from build123d import *

# Parameters (mm, degrees)
SKETCH013_R     = 13
SKETCH013_R_2   = 8.5
PAD008_DEPTH    = 5
SKETCH014_R     = 12
SKETCH014_R_2   = 9.5
POCKET006_DEPTH = 0.5
SKETCH015_R     = 12
SKETCH015_R_2   = 9.5
POCKET007_DEPTH = 0.5


with BuildPart() as part:
    # Sketch013 → Pad008 (new body)
    with BuildSketch(Plane.XY):
        Circle(SKETCH013_R)
        Circle(SKETCH013_R_2, mode=Mode.SUBTRACT)
    extrude(amount=PAD008_DEPTH)

    # Sketch014 → Pocket006 (cut)
    with BuildSketch(Plane.XY.offset(5)):
        Circle(SKETCH014_R)
        Circle(SKETCH014_R_2, mode=Mode.SUBTRACT)
    extrude(amount=-POCKET006_DEPTH, mode=Mode.SUBTRACT)

    # Sketch015 → Pocket007 (cut)
    with BuildSketch(Plane.XY):
        Circle(SKETCH015_R)
        Circle(SKETCH015_R_2, mode=Mode.SUBTRACT)
    extrude(amount=POCKET007_DEPTH, mode=Mode.SUBTRACT)


solid = part.part
Geometry check sheet. Reference: the model listing, model coordinates, mm. A direction names the side the tool comes from. Give positions to 0.01 mm unless a question says otherwise; leave off trailing zeros. Order: outer loops, then holes, each group sorted by start corner. A loop starts at its lowest first (then second) coordinate and runs counter-clockwise, first axis right, second up.
1) Cross-section at C-C (z = 2.65). Record the boundary of the cut face in (x, y).
Results are:
outline: circle Ø26 at (0, 0); hole circle Ø17 at (0, 0)
2) Tool access check on faces 1 (the flat face through (9, 4, 0.5)), 2 (the flat face through (9, 4, 4.5)), 3 (the cylindrical face through (4.57, 7.167, 2.465)). Record the directions out of +Z, -Z, +X, -X, +Y, -Y that give a thin tool (end or side, any length) a straight path to the whole face; none if there is none.
Results are:
face 1: -Z
face 2: +Z
face 3: +Z, -Z
3) Cross-section at A-A (y = 0). Record the boundary of the cut face in (x, z).
Results are:
outline: (-13, 0) - (-12, 0) - (-12, 0.5) - (-9.5, 0.5) - (-9.5, 0) - (-8.5, 0) - (-8.5, 5) - (-9.5, 5) - (-9.5, 4.5) - (-12, 4.5) - (-12, 5) - (-13, 5) - close; (8.5, 0) - (9.5, 0) - (9.5, 0.5) - (12, 0.5) - (12, 0) - (13, 0) - (13, 5) - (12, 5) - (12, 4.5) - (9.5, 4.5) - (9.5, 5) - (8.5, 5) - close
4) Material ranges on probe 1 along Y at (x, z) = (0, 0.35); probe 2 along Y at (x, z) = (0, 2.85); probe 3 along X at (y, z) = (-6, 0.4), recorded low to high.
Results are:
probe 1: y = -13 to -12, -9.5 to -8.5, 8.5 to 9.5, 12 to 13
probe 2: y = -13 to -8.5, 8.5 to 13
probe 3: x = -11.53 to -10.39, -7.37 to -6.02, 6.02 to 7.37, 10.39 to 11.53
5) Gauge pin test, flat ends, axial feed: pin 1 (5 mm diameter, centred on x = -3, y = 7, fed in from +Z); pin 2 (12 mm diameter, centred on x = 1.5, y = 0, fed in from -Z); pin 3 (1 mm diameter, centred on x = -9, z = 2.5, fed in from -Y). Record the tip position at first contact, or that the pin passes through.
Results are:
pin 1: stops at z = 5
pin 2: passes through
pin 3: stops at y = -9.84
6) Cross-section at D-D (x = 11.25). Record the boundary of the cut face in (y, z).
Results are:
outline: (-6.51, 0) - (-4.18, 0) - (-4.18, 0.5) - (4.18, 0.5) - (4.18, 0) - (6.51, 0) - (6.51, 5) - (4.18, 5) - (4.18, 4.5) - (-4.18, 4.5) - (-4.18, 5) - (-6.51, 5) - close
7) Draft check along Y on faces 4 (the flat face through (9, -9, 0)), 5 (the cylindrical face through (4.38, -8.43, 0.25)), 6 (the cylindrical face through (-10.316, -7.91, 2.465)). Enter one of: released by +Y, released by -Y, zero draft, split by the parting line, or undercut.
Results are:
face 4: zero draft
face 5: undercut
face 6: split by the parting line
8) Cross-section at B-B (x = 8). Record the boundary of the cut face in (y, z), then the cut area to 3 significant figures.
Results are:
outline: (-10.25, 0) - (-8.94, 0) - (-8.94, 0.5) - (-5.12, 0.5) - (-5.12, 0) - (-2.87, 0) - (-2.87, 5) - (-5.12, 5) - (-5.12, 4.5) - (-8.94, 4.5) - (-8.94, 5) - (-10.25, 5) - close; (2.87, 0) - (5.12, 0) - (5.12, 0.5) - (8.94, 0.5) - (8.94, 0) - (10.25, 0) - (10.25, 5) - (8.94, 5) - (8.94, 4.5) - (5.12, 4.5) - (5.12, 5) - (2.87, 5) - close
area: 66.1 mm2
